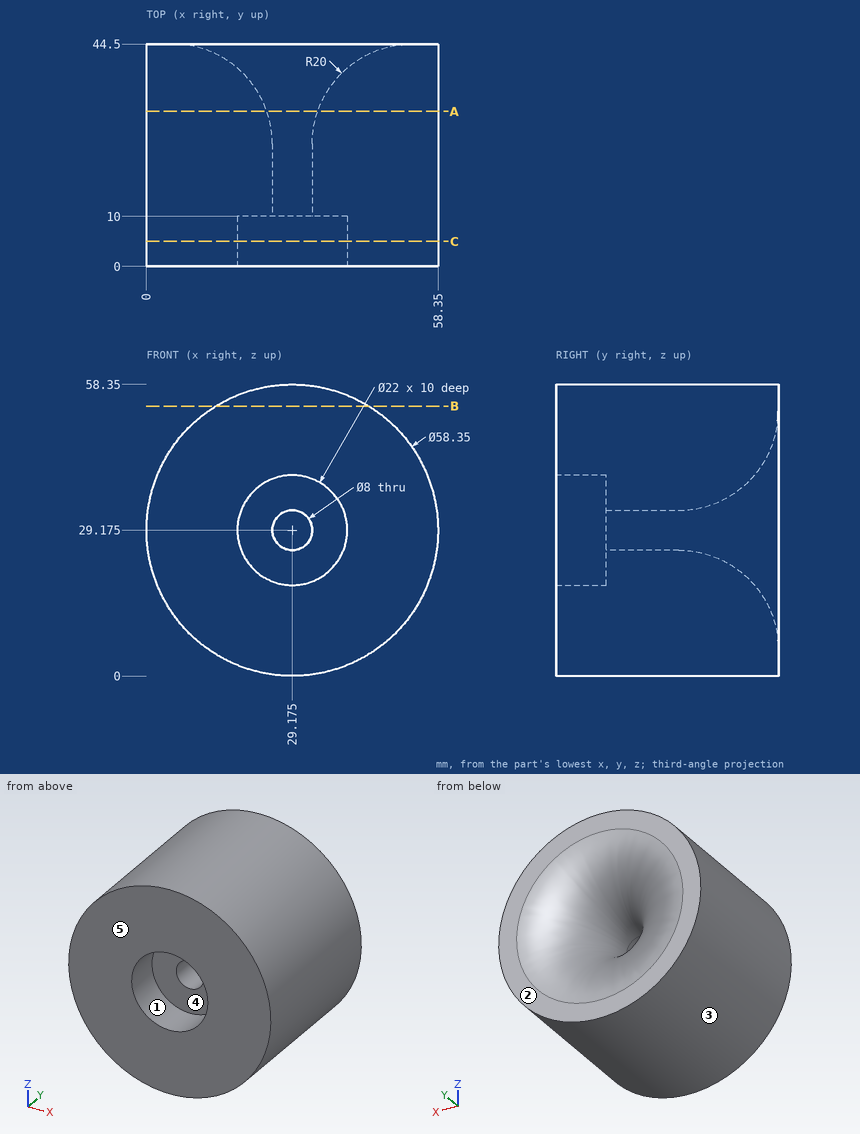
Can you work these out from the drawing? Everything is in mm from the part's minimum corner. A direction names the side the tool comes from. Round coordinates to 2 decimals unless told otherwise and drop trailing zeros. Loops run counter-clockwise (first coordinate to the right, second up) from the corner with the lowest first, then second, coordinate; pieces in that order, holes last. Notation, with made-up numbers: (23.5, 43) -> (60.5, 43) arc R10 cw to (60.5, 51) -> close; hole circle Ø10 at (-12, 3). An arc over 180 degrees is marked (long way). Answer in a Markdown table with one row per item.
Item 1: If I drill on probe 1 along Z at (x, y) = (30.5, 25); probe 2 along X at (y, z) = (34, 31); probe 3 along X at (y, z) = (7, 37.5), over which ranges is the centre line in solid material (lowest first)?
Answer block:
| item | result |
|---|---|
| probe 1 | 0.03 to 25.39, 32.96 to 58.32 |
| probe 2 | 0.06 to 23.04, 35.31 to 58.29 |
| probe 3 | 1.21 to 21.99, 36.36 to 57.14 |
Item 2: On a 3-axis mill with a long thin cutter (end or side, diameter ignored), from which of +Z, -Z, +X, -X, +Y, -Y can I reach the whole of each face in a straight line? I mean the marked faces 1 and 2. Say none if no direction works.
Answer block:
| item | result |
|---|---|
| face 1 | -Y |
| face 2 | +Z, -Z, +X, -X, +Y |
Item 3: Suppose I cut it at B-B, the plane z = 54. List the corners of the cut face in (x, y) for me.
Answer block:
| item | result |
|---|---|
| outline | (13.85, 0) -> (44.5, 0) -> (44.5, 44.5) -> (13.85, 44.5) -> close |
Item 4: Suppose I cut it at A-A, the plane y = 31. List the corners of the cut face in (x, z) for me (3 decimals).
Answer block:
| item | result |
|---|---|
| outline | circle Ø58.35 at (29.175, 29.175); hole circle Ø10.171 at (29.175, 29.175) |
Item 5: We'd pull the mould along X, two halves only. Please class the marked faces 3, 4 and 5: released by +X, released by -X, zero draft, split by the parting line, or undercut.
Answer block:
| item | result |
|---|---|
| face 3 | split by the parting line |
| face 4 | undercut |
| face 5 | zero draft |
Item 6: Suppose I cut it at C-C, the plane y = 5. List the corners of the cut face in (x, z) for me (3 decimals).
Answer block:
| item | result |
|---|---|
| outline | circle Ø58.35 at (29.175, 29.175); hole circle Ø22 at (29.175, 29.175) |
Item 7: Will these pins go through, and if not, where does the flat tip stop? P1, Ø10, axis at y = 12, z = 33.5, coming from the -X side; P2, Ø2, axis at x = 22, y = 5.5, coming from the +Z side; P3, Ø5, axis at x = 35.5, z = 30, coming from the -Y side; P4, Ø1, axis at x = 13.5, z = 39, coming from the -Y side.
Answer block:
| item | result |
|---|---|
| P1 | x = 0 |
| P2 | z = 57.69 |
| P3 | y = 10 |
| P4 | y = 0 |
